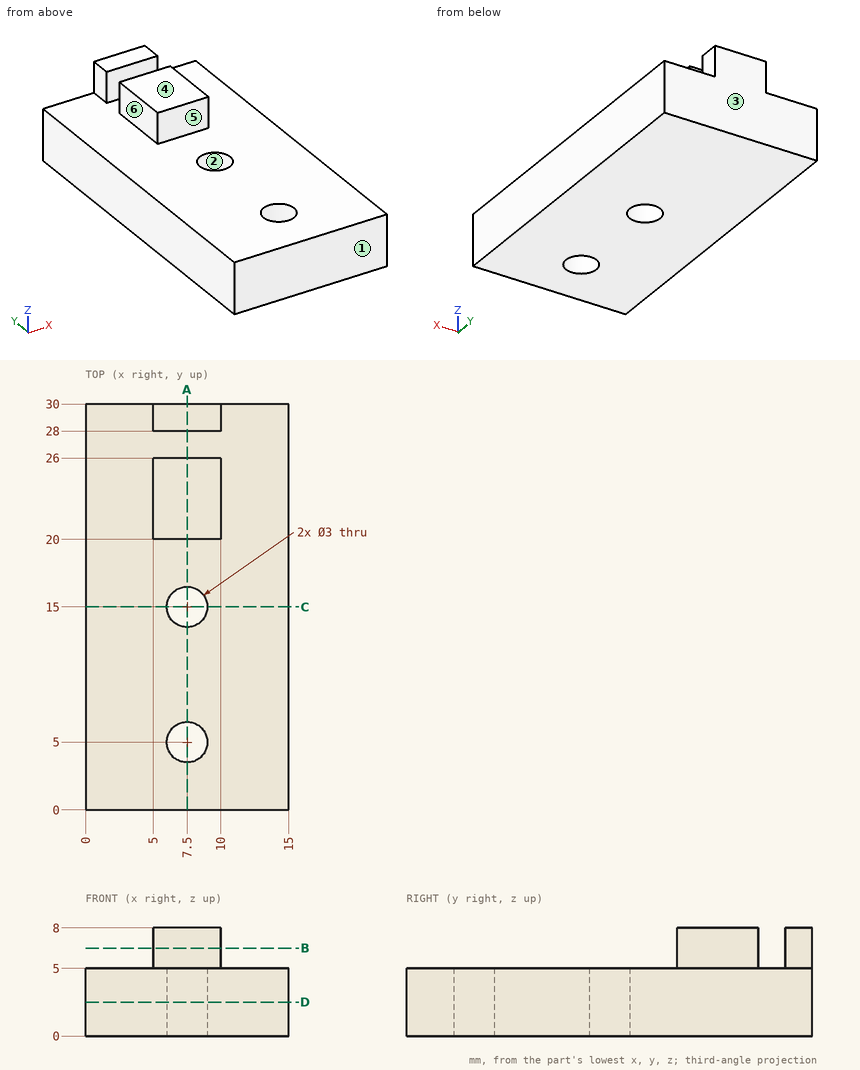
Job drawing, mm, ordinate dimensions from the low corner. One solid piece. A direction names the side the tool comes from. Give positions to 0.01 mm unless a question says otherwise; leave off trailing zeros. Order: outer loops, then holes, each group sorted by start corner. A loop starts at its lowest first (then second) coordinate and runs counter-clockwise, first axis right, second up. Notation, with made-up numbers: (-1, 58) - (31, 58) arc R30 cw to (31, 80) - close; hole circle Ø9 at (76.25, 4.25). An arc over 180 degrees is marked (long way). Return JSON: item names as keys, results as strings.
1) 3-axis set-ups, long thin cutter, end or side, ignore diameter. For the marked faces 4, 5 and 6: which of +Z, -Z, +X, -X, +Y, -Y reach the whole face in a straight line?
Geometry says:
{"face 4": "+Z, +X, -X, +Y, -Y", "face 5": "+Z, +X, -X, -Y", "face 6": "+Z, -X, +Y, -Y"}
2) Cut at B-B, the plane z = 6.5. Give the cut face in (x, y), plus the area to 3 significant figures.
Geometry says:
{"outline": "(5, 20) - (10, 20) - (10, 26) - (5, 26) - close; (5, 28) - (10, 28) - (10, 30) - (5, 30) - close", "area": "40.0 mm²"}
3) Cut at C-C, the plane y = 15. Give the cut face in (x, z), plus the area to 3 significant figures.
Geometry says:
{"outline": "(0, 0) - (6, 0) - (6, 5) - (0, 5) - close; (9, 0) - (15, 0) - (15, 5) - (9, 5) - close", "area": "60.0 mm²"}
4) Cut at D-D, the plane z = 2.5. Give the cut face in (x, y), plus the area to 3 significant figures.
Geometry says:
{"outline": "(0, 0) - (15, 0) - (15, 30) - (0, 30) - close; hole circle Ø3 at (7.5, 5); hole circle Ø3 at (7.5, 15)", "area": "436 mm²"}
5) Flat gauge pins, fed straight in: P1, Ø3.5, axis at y = 24, z = 7, coming from the -X side; P2, Ø0.6, axis at y = 29.5, z = 7, coming from the +X side; P3, Ø1.8, axis at x = 7.5, y = 5, coming from the +Z side. Where does each tip first touch, or does it go through?
Geometry says:
{"P1": "x = 5", "P2": "x = 10", "P3": "through"}
6) Probe line 1 (Y direction, x = 7.5, z = 2.4); line 2 (X direction, y = 15, z = 3.45); line 3 (Z direction, x = 10.25, y = 5). List the from-to ranges inside material, lowest first. Write a range as from..to.
Geometry says:
{"line 1": "0..3.5, 6.5..13.5, 16.5..30", "line 2": "0..6, 9..15", "line 3": "0..5"}
7) Pull direction Y, two halves, no side cores. Call the marked faces 1, 2 and 3: pulls with the +Y half, pulls with the -Y half, needs draft (parallel to the pull), parting line crosses it, or undercut.
Geometry says:
{"face 1": "pulls with the -Y half", "face 2": "undercut", "face 3": "pulls with the +Y half"}
8) Cut at A-A, the plane x = 7.5. Give the cut face in (y, z), plus the area to 3 significant figures.
Geometry says:
{"outline": "(0, 0) - (3.5, 0) - (3.5, 5) - (0, 5) - close; (6.5, 0) - (13.5, 0) - (13.5, 5) - (6.5, 5) - close; (16.5, 0) - (30, 0) - (30, 8) - (28, 8) - (28, 5) - (26, 5) - (26, 8) - (20, 8) - (20, 5) - (16.5, 5) - close", "area": "144 mm²"}
